Solid Edge part; units mm, degrees
sketch "Sketch1" plane through (0, 0, 0) normal (0, -1, 0) x (1, 0, 0)
  line L0 (55.0871, 62.6934) -> (55.0871, 40.6934)
  line L1 (55.0871, 40.6934) -> (157.0871, 40.6934)
  line L2 (157.0871, 40.6934) -> (157.0871, 62.6934)
  line L3 (157.0871, 62.6934) -> (55.0871, 62.6934)
  dimension "D1" = 55.0871
extrude "Protrusion1" add sketch "Sketch1" against normal blind 15
sketch "Sketch2" plane through (106.0871, 7.5, 62.6934) normal (0, 0, 1) x (1, 0, 0)
  circle A0 centre (-46, 0) radius 2
  circle A1 centre (-37, 0) radius 2
  circle A2 centre (45, 0) radius 2
extrude "Cutout1" cut sketch "Sketch2" against normal through all
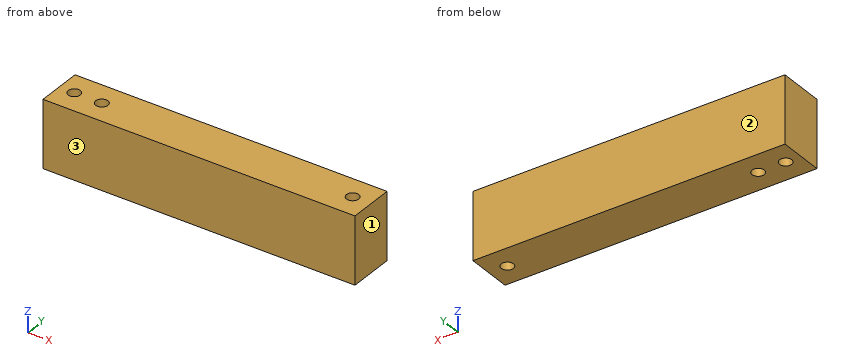
Model file for the job. Use its own axes, mm. Face numbers are marked on the shaded views. Round coordinates to 2 decimals unless told otherwise and drop trailing zeros. Write each loop counter-clockwise with the first axis right and the second up, starting at its lowest first coordinate (ties: lowest second). Pieces come first, ordered by that corner, then holes. Notation, with made-up numbers: (-23.5, 22.25) - (-19.5, 22.25) arc R25 ccw to (-19.5, 54.25) - close; hole circle Ø2 at (50, 78.5). An arc over 180 degrees is marked (long way). One line per item, written item: value.
(1) Cut at B-B, the plane y = 7.5. Give the cut face in (x, z), plus the area to 3 significant figures.
Values follow:
outline: (55.09, 40.69) - (58.09, 40.69) - (58.09, 62.69) - (55.09, 62.69) - close; (62.09, 40.69) - (67.09, 40.69) - (67.09, 62.69) - (62.09, 62.69) - close; (71.09, 40.69) - (149.09, 40.69) - (149.09, 62.69) - (71.09, 62.69) - close; (153.09, 40.69) - (157.09, 40.69) - (157.09, 62.69) - (153.09, 62.69) - close
area: 1,980 mm²
(2) Two-plate mould, pull along Y, no slides. Class the marked faces 1, 2 and 3: pulls with the +Y half, pulls with the -Y half, needs draft (parallel to the pull), parting line crosses it, or undercut.
Values follow:
face 1: needs draft
face 2: pulls with the +Y half
face 3: pulls with the -Y half
(3) Cut at A-A, the plane z = 56.5. Give the cut face in (x, y).
Values follow:
outline: (55.09, 0) - (157.09, 0) - (157.09, 15) - (55.09, 15) - close; hole circle Ø4 at (60.09, 7.5); hole circle Ø4 at (69.09, 7.5); hole circle Ø4 at (151.09, 7.5)
(4) Drop a flat-ended pin along its axis: P1, Ø2.5, axis at x = 69.09, y = 7.5, coming from the +Z side. Give the stop position or say it passes through.
Values follow:
P1: passes through
(5) Wall check: probe 1 along X at (y, z) = (6.5, 54); probe 2 along Y at (x, z) = (68.5, 53.75). Give the ranges that are in metal, low to high.
Values follow:
probe 1: x = 55.09 to 58.36, 61.82 to 67.36, 70.82 to 149.36, 152.82 to 157.09
probe 2: y = 0 to 5.59, 9.41 to 15
